```python
from build123d import *

# Parameters (mm, degrees)
SKETCH_1_R          = 1.5
EXTRUDE_1_DEPTH     = 5
CHAMFER_1_SIZE      = 5
SKETCH_3_R          = 1.5
CUT_EXTRUDE_2_DEPTH = 10
FILLET_1_R          = 10
FILLET_2_R          = 2
CUT_EXTRUDE_3_DEPTH = 199.053023203
EXTRUDE_2_DEPTH     = 5


with BuildPart() as part:
    # 草图1 → 凸台-拉伸1 (new body)
    with BuildSketch(Plane.XY):
        Polygon((-100, -140), (-100, -60), (-140, -60), (-140, 60), (-100, 60), (-100, 140), (100, 140), (100, 60), (140, 60), (140, -60), (100, -60), (100, -140), align=None)
        with Locations((-40, -130)):
            Circle(SKETCH_1_R, mode=Mode.SUBTRACT)
        with Locations((-40, -35)):
            Circle(SKETCH_1_R, mode=Mode.SUBTRACT)
        with Locations(Location((40, -130, 0), (0, 0, 180))):
            Circle(SKETCH_1_R, mode=Mode.SUBTRACT)
        with Locations(Location((40, -35, 0), (0, 0, 180))):
            Circle(SKETCH_1_R, mode=Mode.SUBTRACT)
        with Locations(Location((-40, 130, 0), (0, 0, 180))):
            Circle(SKETCH_1_R, mode=Mode.SUBTRACT)
        with Locations((40, 130)):
            Circle(SKETCH_1_R, mode=Mode.SUBTRACT)
        with Locations((40, 35)):
            Circle(SKETCH_1_R, mode=Mode.SUBTRACT)
        with Locations(Location((-40, 35, 0), (0, 0, 180))):
            Circle(SKETCH_1_R, mode=Mode.SUBTRACT)
        with Locations((-39, 39)):
            Circle(SKETCH_1_R, mode=Mode.SUBTRACT)
        with Locations((39, 39)):
            Circle(SKETCH_1_R, mode=Mode.SUBTRACT)
        with Locations((39, -39)):
            Circle(SKETCH_1_R, mode=Mode.SUBTRACT)
        with Locations((-39, -39)):
            Circle(SKETCH_1_R, mode=Mode.SUBTRACT)
    extrude(amount=EXTRUDE_1_DEPTH)

    # 倒角1
    chamfer_1_edges = [part.edges().sort_by_distance(p)[0] for p in [
        (-100, -140, 2.5),
        (-100, -60, 2.5),
        (-140, -60, 2.5),
        (-140, 60, 2.5),
        (-100, 60, 2.5),
        (-100, 140, 2.5),
        (100, 140, 2.5),
        (100, 60, 2.5),
        (140, 60, 2.5),
        (140, -60, 2.5),
        (100, -60, 2.5),
        (100, -140, 2.5),
    ]]
    chamfer(chamfer_1_edges, length=CHAMFER_1_SIZE)

    # 草图3 → 切除-拉伸2 (cut)
    with BuildSketch(Plane.XY.offset(5)):
        with Locations((-88, 135)):
            Circle(SKETCH_3_R)
        with Locations((-58, 135)):
            Circle(SKETCH_3_R)
        with Locations((58, 135)):
            Circle(SKETCH_3_R)
        with Locations((88, 135)):
            Circle(SKETCH_3_R)
        with Locations((88, -135)):
            Circle(SKETCH_3_R)
        with Locations((58, -135)):
            Circle(SKETCH_3_R)
        with Locations((-58, -135)):
            Circle(SKETCH_3_R)
        with Locations((-88, -135)):
            Circle(SKETCH_3_R)
        with Locations((-80, 0)):
            Circle(SKETCH_3_R)
        with Locations((-69.282032303, 40)):
            Circle(SKETCH_3_R)
        with Locations((69.282032303, 40)):
            Circle(SKETCH_3_R)
        with Locations((80, 0)):
            Circle(SKETCH_3_R)
        with Locations((69.282032303, -40)):
            Circle(SKETCH_3_R)
        with Locations((-69.282032303, -40)):
            Circle(SKETCH_3_R)
        with BuildLine():
            Line((-25, -35), (25, -35))
            ThreePointArc((25, -35), (29.393398282, -45.606601718), (40, -50))
            Line((40, -50), (40, -115))
            ThreePointArc((40, -115), (29.393398282, -119.393398282), (25, -130))
            Line((25, -130), (-25, -130))
            ThreePointArc((-25, -130), (-29.393398282, -119.393398282), (-40, -115))
            Line((-40, -115), (-40, -50))
            ThreePointArc((-40, -50), (-29.393398282, -45.606601718), (-25, -35))
        make_face()
        with BuildLine():
            Line((-25, 35), (25, 35))
            ThreePointArc((25, 35), (29.393398282, 45.606601718), (40, 50))
            Line((40, 50), (40, 115))
            ThreePointArc((40, 115), (29.393398282, 119.393398282), (25, 130))
            Line((25, 130), (-25, 130))
            ThreePointArc((-25, 130), (-29.393398282, 119.393398282), (-40, 115))
            Line((-40, 115), (-40, 50))
            ThreePointArc((-40, 50), (-29.393398282, 45.606601718), (-25, 35))
        make_face()
        Polygon((-20.071531448, -8.109425098), (-8.458486518, -19.926945474), (8.109425098, -20.071531448), (19.926945474, -8.458486518), (20.071531448, 8.109425098), (8.458486518, 19.926945474), (-8.109425098, 20.071531448), (-19.926945474, 8.458486518), align=None)
        Polygon((-107.5, 40), (-82.5, 40), (-82.5, 28), (-95.5, 28), (-103, 20.5), (-103, -20.5), (-95.5, -28), (-82.5, -28), (-82.5, -40), (-107.5, -40), (-115, -32.5), (-115, 32.5), align=None)
        Polygon((107.5, -40), (82.5, -40), (82.5, -28), (95.5, -28), (103, -20.5), (103, 20.5), (95.5, 28), (82.5, 28), (82.5, 40), (107.5, 40), (115, 32.5), (115, -32.5), align=None)
        with BuildLine():
            ThreePointArc((-73, -85), (-80.5, -92.5), (-73, -100))
            ThreePointArc((-73, -100), (-65.5, -107.5), (-73, -115))
            ThreePointArc((-73, -115), (-88, -100), (-73, -85))
        make_face()
        with BuildLine():
            ThreePointArc((-73, 85), (-88, 100), (-73, 115))
            ThreePointArc((-73, 115), (-65.5, 107.5), (-73, 100))
            ThreePointArc((-73, 100), (-80.5, 92.5), (-73, 85))
        make_face()
        with BuildLine():
            ThreePointArc((73, -85), (88, -100), (73, -115))
            ThreePointArc((73, -115), (65.5, -107.5), (73, -100))
            ThreePointArc((73, -100), (80.5, -92.5), (73, -85))
        make_face()
        with BuildLine():
            ThreePointArc((73, 85), (80.5, 92.5), (73, 100))
            ThreePointArc((73, 100), (65.5, 107.5), (73, 115))
            ThreePointArc((73, 115), (88, 100), (73, 85))
        make_face()
    extrude(amount=-CUT_EXTRUDE_2_DEPTH, mode=Mode.SUBTRACT)

    # 圆角1
    fillet_1_edges = [part.edges().sort_by_distance(p)[0] for p in [
        (-25, 35, 2.5),
        (-40, 50, 2.5),
        (-40, 115, 2.5),
        (-25, 130, 2.5),
        (25, 130, 2.5),
        (40, 115, 2.5),
        (40, 50, 2.5),
        (25, 35, 2.5),
        (-25, -130, 2.5),
        (-40, -115, 2.5),
        (-40, -50, 2.5),
        (-25, -35, 2.5),
        (25, -35, 2.5),
        (40, -50, 2.5),
        (40, -115, 2.5),
        (25, -130, 2.5),
    ]]
    fillet(fillet_1_edges, radius=FILLET_1_R)

    # 圆角2
    fillet_2_edges = [part.edges().sort_by_distance(p)[0] for p in [
        (-82.5, -40, 2.5),
        (-107.5, -40, 2.5),
        (-115, -32.5, 2.5),
        (-115, 32.5, 2.5),
        (-107.5, 40, 2.5),
        (-82.5, 40, 2.5),
        (-82.5, 28, 2.5),
        (-95.5, 28, 2.5),
        (-103, 20.5, 2.5),
        (-103, -20.5, 2.5),
        (-95.5, -28, 2.5),
        (-82.5, -28, 2.5),
        (115, -32.5, 2.5),
        (107.5, -40, 2.5),
        (82.5, -40, 2.5),
        (82.5, -28, 2.5),
        (95.5, -28, 2.5),
        (103, -20.5, 2.5),
        (103, 20.5, 2.5),
        (95.5, 28, 2.5),
        (82.5, 28, 2.5),
        (82.5, 40, 2.5),
        (107.5, 40, 2.5),
        (115, 32.5, 2.5),
    ]]
    fillet(fillet_2_edges, radius=FILLET_2_R)

    # 草图5 → 切除-拉伸3 (cut, through all)
    with BuildSketch(Plane.XY.offset(5)):
        Polygon((0, -140), (0, 140), (-95, 140), (-100, 135), (-100, 65), (-105, 60), (-135, 60), (-140, 55), (-140, -55), (-135, -60), (-105, -60), (-100, -65), (-100, -135), (-95, -140), align=None)
    extrude(amount=-CUT_EXTRUDE_3_DEPTH, mode=Mode.SUBTRACT)

    # 草图6 → 凸台-拉伸2 (add)
    with BuildSketch(Plane(origin=(0, 0, 0), x_dir=(-1, 0, 0), z_dir=(0, 0, -1))):
        with BuildLine():
            Line((0, 35), (0, 130))
            Line((0, 130), (-17.087121525, 130))
            ThreePointArc((-17.087121525, 130), (-22.5643471, 128.366600265), (-26.252272915, 124))
            ThreePointArc((-26.252272915, 124), (-29.393398282, 119.393398282), (-34, 116.252272915))
            ThreePointArc((-34, 116.252272915), (-38.366600265, 112.5643471), (-40, 107.087121525))
            Line((-40, 107.087121525), (-40, 57.912878475))
            ThreePointArc((-40, 57.912878475), (-38.366600265, 52.4356529), (-34, 48.747727085))
            ThreePointArc((-34, 48.747727085), (-29.393398282, 45.606601718), (-26.252272915, 41))
            ThreePointArc((-26.252272915, 41), (-22.5643471, 36.633399735), (-17.087121525, 35))
            Line((-17.087121525, 35), (0, 35))
        make_face()
        Polygon((0, -20.000761568), (0, 20.000761568), (-8.458486518, 19.926945474), (-20.071531448, 8.109425098), (-19.926945474, -8.458486518), (-8.109425098, -20.071531448), align=None)
        with BuildLine():
            Line((0, -130), (0, -35))
            Line((0, -35), (-17.087121525, -35))
            ThreePointArc((-17.087121525, -35), (-22.5643471, -36.633399735), (-26.252272915, -41))
            ThreePointArc((-26.252272915, -41), (-29.393398282, -45.606601718), (-34, -48.747727085))
            ThreePointArc((-34, -48.747727085), (-38.366600265, -52.4356529), (-40, -57.912878475))
            Line((-40, -57.912878475), (-40, -107.087121525))
            ThreePointArc((-40, -107.087121525), (-38.366600265, -112.5643471), (-34, -116.252272915))
            ThreePointArc((-34, -116.252272915), (-29.393398282, -119.393398282), (-26.252272915, -124))
            ThreePointArc((-26.252272915, -124), (-22.5643471, -128.366600265), (-17.087121525, -130))
            Line((-17.087121525, -130), (0, -130))
        make_face()
    extrude(amount=-EXTRUDE_2_DEPTH)


solid = part.part
```
The model under review builds one solid part; all positions refer to its coordinate system, in mm. A direction names the side the tool comes from. Coordinates: 2 decimals unless noted, no trailing zeros. Write each loop counter-clockwise with the first axis right and the second up, starting at its lowest first coordinate (ties: lowest second). Pieces come first, ordered by that corner, then holes. Notation, with made-up numbers: (-2, -2) - (37, -2) arc R22 ccw to (37, 9) - close; hole circle Ø8 at (25, 51). An arc over 180 degrees is marked (long way). Answer in a Markdown table with one row per item. Add a question column.
Q1. Consider section B-B on z = 1.1. Give the number of separate pieces and of enclosed holes in the cut face, then the cut area to 3 significant figures.
Q2. For faces 1 (the face through (120, 60, 2)), 2 (the face through (0, -2, 2)), 3 (the face through (120, -60, 2)), 4 (the face through (115, 0, 3)), list the 3-axis set-ups (+Z, -Z, +X, -X, +Y, -Y) from which the entire face can be reached by the end or side of a thin tool; tool diameter is ignored.
Q3. Clearance check with flat-ended pins moving along their axes: pin 1 (2 mm diameter, centred on y = 80.5, z = 3.5, fed in from +X); pin 2 (1.5 mm diameter, centred on x = 125.5, z = 2, fed in from -Y). State where each tip first meets the part, or that it passes through.
Q4. Draft analysis for pull direction Y (two halves, no side actions). For faces 5 (the face through (98, 137, 2)), 6 (the face through (82.5, -34, 3)), 7 (the face through (140, 1, 2)), state which applies: +Y half, -Y half, draft (parallel to the pull), parting line (faces both ways), or undercut.
Q5. To check wall thickness, follow line 1 along X through (y, z) = (-135, 2.4); line 2 along Y through (x, z) = (72.5, 1.75); line 3 along Y through (x, z) = (127, 0.85). State the ranges of each line that lie inside material, in increasing order. Write a range as from..to.
Q6. Consider section A-A on y = 107.5. Give the boundary of the cut face in (x, z).
Q7. Consider section C-C on y = -92.5. Give the boundary of the cut face in (x, z), then the cut area to 3 significant figures.
Q8. Consider section D-D on y = 71.5. Give the boundary of the cut face in (x, z).
Answers below:
| question | item | result |
|---|---|---|
| 1 | separate pieces | 1 |
| 1 | enclosed holes | 16 |
| 1 | area | 30,500 mm² |
| 2 | face 1 | +Z, -Z, +X, +Y |
| 2 | face 2 | +Z, -Z, -X, +Y, -Y |
| 2 | face 3 | +Z, -Z, +X, -Y |
| 2 | face 4 | +Z, -Z |
| 3 | pin 1 | x = 100 |
| 3 | pin 2 | y = -60 |
| 4 | face 5 | +Y half |
| 4 | face 6 | undercut |
| 4 | face 7 | draft |
| 5 | line 1 | 0..56.5, 59.5..86.5, 89.5..100 |
| 5 | line 2 | -140..-114.98, -100.02..100.02, 114.98..140 |
| 5 | line 3 | -60..60 |
| 6 | outline | (0, 0) - (65.5, 0) - (65.5, 5) - (0, 5) - close; (85.99, 0) - (100, 0) - (100, 5) - (85.99, 5) - close |
| 7 | outline | (0, 0) - (80.5, 0) - (80.5, 5) - (0, 5) - close; (85.99, 0) - (100, 0) - (100, 5) - (85.99, 5) - close |
| 7 | area | 473 mm² |
| 8 | outline | (0, 0) - (100, 0) - (100, 5) - (0, 5) - close |
